```python
from build123d import *

# Parameters (mm, degrees)
SKETCH_W  = 90
SKETCH_H  = 60
PAD_DEPTH = 2


with BuildPart() as pad:
    # Sketch → Pad (new body)
    with BuildSketch(Plane.XY):
        with Locations((15, 0)):
            Rectangle(SKETCH_W, SKETCH_H)
    extrude(amount=PAD_DEPTH)


with BuildPart() as cone:
    # Cone → Cone (revolve)
    with BuildSketch(Plane.XZ):
        Polygon((0, 0), (19.5, 0), (27, 15), (0, 15), align=None)
    revolve(axis=Axis((0, 0, 0), (0, 0, 1)))


with BuildPart() as fusion:
    # Cone001 → Cone001 (revolve)
    with BuildSketch(Plane.XZ):
        Polygon((0, 0), (21, 0), (29, 15), (0, 15), align=None)
    revolve(axis=Axis((0, 0, 0), (0, 0, 1)))

    # Cut: cut Cone
    add(cone.part, mode=Mode.SUBTRACT)


with BuildPart() as fusion_1:
    # Cut placement: moved
    add(fusion.part.moved(Location((0, 0, 2))))

    # Fusion: union Pad
    add(pad.part)


solid = fusion_1.part
```
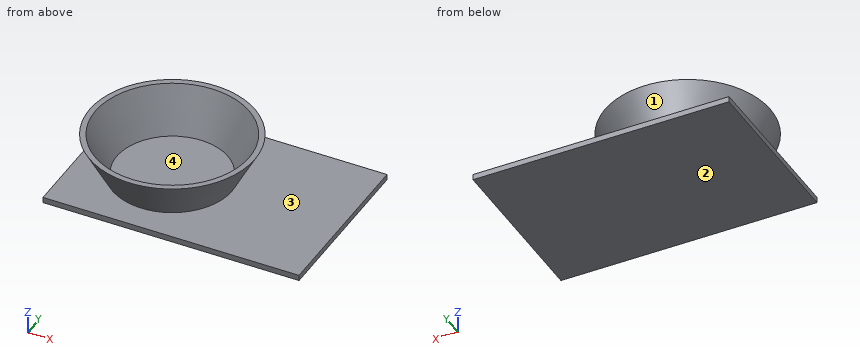
Geometry: final body of the model. Coordinates: model frame, mm. Face numbers are marked on the shaded views. A direction names the side the tool comes from. Coordinates: 2 decimals unless noted, no trailing zeros. Order: outer loops, then holes, each group sorted by start corner. A loop starts at its lowest first (then second) coordinate and runs counter-clockwise, first axis right, second up. Notation, with made-up numbers: M 86,14 L 132,14 A20 ccw 132,20 Z; hole C -36,-39.5 d6. An arc over 180 degrees is marked long. Answer in a Markdown table with one row per item. Add a question column.
Q1. Mould query, pull axis X, two halves, no side actions, for the marked faces 3 and 4. Classes: released by +X, released by -X, zero draft, split by the parting line, or undercut.
Q2. Line query: L1, parallel to Z at x = 32, y = -12; L2, parallel to Z at x = -12.5, y = -21.5; L3, parallel to X at y = 22, z = 13. Output: solid intervals per line, ascending.
Q3. Section query B-B on y = 0. Return the cut outline in (x, z), and give its area (4 significant figures).
Q4. Section query C-C on z = 12.5. Return the cut outline in (x, y), and give its area (3 significant figures).
Q5. Contact query for flat-ended pins moving along their axis: P1, Ø12, axis at x = 7.5, y = 18.5, coming from the +Z side; P2, Ø1.5, axis at x = 20, y = 5, coming from the +Z side; P3, Ø3, axis at y = 19, z = 4.5, coming from the +X side. Output: stop coordinate, or through.
Q6. Section query D-D on x = 49. Return the cut outline in (y, z), and give its area (3 significant figures).
Q7. Section query A-A on x = 0. Return the cut outline in (y, z).
Q8. Reachability of the marked faces 1 and 2 from +Z, -Z, +X, -X, +Y, -Y: full face, straight path, thin tool, end or side. Return the list, or none.
Completed:
| question | item | result |
|---|---|---|
| 1 | face 3 | zero draft |
| 1 | face 4 | undercut |
| 2 | L1 | z = 0 to 2 |
| 2 | L2 | z = 0 to 2, 9.26 to 12.74 |
| 2 | L3 | x = -15.42 to -11.87, 11.87 to 15.42 |
| 3 | outline | M -30,0 L 60,0 L 60,2 L 21,2 L 29,17 L 27,17 L 19.5,2 L -19.5,2 L -27,17 L -29,17 L -21,2 L -30,2 Z |
| 3 | area | 232.5 mm2 |
| 4 | outline | C 0,0 d53.2; hole C 0,0 d49.5 |
| 4 | area | 298 mm2 |
| 5 | P1 | stops at z = 14.92 |
| 5 | P2 | stops at z = 5.73 |
| 5 | P3 | stops at x = 14.27 |
| 6 | outline | M -30,0 L 30,0 L 30,2 L -30,2 Z |
| 6 | area | 120 mm2 |
| 7 | outline | M -30,0 L 30,0 L 30,2 L 21,2 L 29,17 L 27,17 L 19.5,2 L -19.5,2 L -27,17 L -29,17 L -21,2 L -30,2 Z |
| 8 | face 1 | none |
| 8 | face 2 | -Z, +X, -X, +Y, -Y |
